Part model, mm, in its own coordinate system. Face numbers are marked on the shaded views. A direction names the side the tool comes from. Coordinates: 2 decimals unless noted, no trailing zeros. Order: outer loops, then holes, each group sorted by start corner. A loop starts at its lowest first (then second) coordinate and runs counter-clockwise, first axis right, second up. Notation, with made-up numbers: (66.25, 22) - (89.25, 22) arc R30 ccw to (89.25, 48) - close; hole circle Ø1 at (38, 72.5). An arc over 180 degrees is marked (long way). Use a Markdown table: item, result. Add a question column.
1) Saw through at A-A on x = 0. List the corners of the cut face in (y, z), then the cut area to 3 significant figures.
2) Drop flat-ended pins along their axis: P1, Ø1.5, axis at y = 41, z = 14.5, coming from the +X side; P2, Ø5.5, axis at x = 22, z = 7, coming from the +Y side; P3, Ø5.5, axis at x = -20, z = 9, coming from the +Y side. Give the stop position or say it passes through.
3) Two-plate mould, pull along Y, no slides. Class the marked faces 1, 2 and 3: +Y half, -Y half, draft (parallel to the pull), parting line (faces both ways), or undercut.
4) Saw through at B-B on y = 26.5. List the corners of the cut face in (x, z).
5) Saw through at C-C on z = 6. Count the separate pieces of the cut face and the enclosed holes in it, then the cut area to 3 significant figures.
6) Wall check: L1, parallel to X at y = 7.75, z = 15.3 (3 decimals); L2, parallel to X at y = 20.5, z = 14.75; L3, parallel to Y at x = 0, z = 9.75. Give the ranges that are in metal, low to high. Write a range as [from, to].
7) Tool access for the marked faces 4 and 5: list every direction of +Z, -Z, +X, -X, +Y, -Y with a clear straight run to the whole face (end or side of a thin tool).
```python
from build123d import *

# Parameters (mm, degrees)
SKETCH_1_R               = 6
EXTRUDE_1_DEPTH          = 18.3
CUT_EXTRUDE_1_DEPTH      = 38
SKETCH_3_R               = 2.15
CUT_EXTRUDE_2_DEPTH      = 74
CUT_EXTRUDE_START        = -74
SKETCH_5_W               = 10
SKETCH_5_H               = 40.552439024
CUT_EXTRUDE_3_DEPTH      = 156.521752466
CUT_EXTRUDE_4_DEPTH      = 40
SKETCH_8_W               = 6
SKETCH_8_H               = 37.346305337
EXTRUDE_2_DEPTH          = 18.3
FILLET_2_R               = 3
FILLET_3_R               = 5
CUT_EXTRUDE_7_DEPTH      = 80
CUT_EXTRUDE_7_DEPTH_BACK = 40
SKETCH_12_R              = 1.525


with BuildPart() as part:
    # 草图1 → 凸台-拉伸1 (new body)
    with BuildSketch(Plane.XY):
        with BuildLine():
            Line((-8.281928864, 111.239451243), (-56, 56.65))
            Line((-56, 56.65), (-56, 0))
            Line((-56, 0), (56, 0))
            Line((56, 0), (56, 56.65))
            Line((56, 56.65), (8.281928864, 111.239451243))
            ThreePointArc((8.281928864, 111.239451243), (0, 115), (-8.281928864, 111.239451243))
        make_face()
        with Locations((0, 104)):
            Circle(SKETCH_1_R, mode=Mode.SUBTRACT)
    extrude(amount=EXTRUDE_1_DEPTH)

    # 草图2 → Cut-Extrude 1 (cut)
    with BuildSketch(Plane.XY.offset(18.3)):
        Polygon((15.622574059, 56.346305337), (56, 36.65), (56, 56.65), (30, 116.346305337), (-30, 116.346305337), (-56, 56.65), (-56, 36.65), (-15.622574059, 56.346305337), align=None)
    extrude(amount=-CUT_EXTRUDE_1_DEPTH, mode=Mode.SUBTRACT)

    # 草图3 → 切除-拉伸2 (cut)
    with BuildSketch(Plane.XY.offset(18.3)):
        with Locations((0, 51.346305337)):
            Circle(SKETCH_3_R)
        with Locations((43, 31.65)):
            Circle(SKETCH_3_R)
        with Locations((43, 5)):
            Circle(SKETCH_3_R)
        with Locations((-43, 5)):
            Circle(SKETCH_3_R)
        with Locations((-43, 31.65)):
            Circle(SKETCH_3_R)
        with Locations((0, 5)):
            Circle(SKETCH_3_R)
    extrude(amount=-CUT_EXTRUDE_2_DEPTH, mode=Mode.SUBTRACT)

    # 草图5 → Cut-Extrude 3 (cut)
    with BuildSketch(Plane.XY.offset(18.3).offset(CUT_EXTRUDE_START)):
        with Locations((53, 20.276219512)):
            Rectangle(SKETCH_5_W, SKETCH_5_H)
    cut_extrude_3 = extrude(amount=CUT_EXTRUDE_3_DEPTH, mode=Mode.SUBTRACT)

    # 镜向2: Cut-Extrude 3 across plane
    add(cut_extrude_3.mirror(Plane(origin=(0, 0, 0), x_dir=(0, 0, 1), z_dir=(1, 0, 0))), mode=Mode.SUBTRACT)

    # 草图7 → 切除-拉伸4 (cut)
    with BuildSketch(Plane(origin=(0, 0, 0), x_dir=(-1, 0, 0), z_dir=(0, 0, -1))):
        Polygon((-38, 34.304151485), (-38, 10), (38, 10), (38, 34.304151485), (11.263584603, 47.346305337), (-11.263584603, 47.346305337), align=None)
    extrude(amount=-CUT_EXTRUDE_4_DEPTH, mode=Mode.SUBTRACT)

    # 草图8 → 凸台-拉伸2 (add)
    with BuildSketch(Plane(origin=(0, 0, 0), x_dir=(-1, 0, 0), z_dir=(0, 0, -1))):
        with Locations((0, 28.673152669)):
            Rectangle(SKETCH_8_W, SKETCH_8_H)
    extrude(amount=-EXTRUDE_2_DEPTH)

    # 圆角2
    fillet_2_edges = [part.edges().sort_by_distance(p)[0] for p in [
        (38, 34.304151485, 9.15),
        (11.263584603, 47.346305337, 9.15),
        (-11.263584603, 47.346305337, 9.15),
        (-38, 34.304151485, 9.15),
        (-38, 10, 9.15),
        (38, 10, 9.15),
        (3, 10, 9.15),
        (-3, 10, 9.15),
        (-3, 47.346305337, 9.15),
        (3, 47.346305337, 9.15),
    ]]
    fillet(fillet_2_edges, radius=FILLET_2_R)

    # 圆角3
    fillet_3_edges = [part.edges().sort_by_distance(p)[0] for p in [
        (-48, 40.552439024, 9.15),
        (-48, 0, 9.15),
        (15.622574059, 56.346305337, 9.15),
        (-15.622574059, 56.346305337, 9.15),
        (48, 40.552439024, 9.15),
        (48, 0, 9.15),
    ]]
    fillet(fillet_3_edges, radius=FILLET_3_R)

    # 草图12 → 切除-拉伸7 (cut, two sides: drawn at the far end of the back side and taken through both)
    with BuildSketch(Plane(origin=(0, 10, 0), x_dir=(1, 0, 0), z_dir=(0, 1, 0)).offset(-CUT_EXTRUDE_7_DEPTH_BACK)):
        with Locations(Location((-10, -15.3, 0), (0, 0, 90))):
            Circle(SKETCH_12_R)
        with Locations(Location((10, -15.3, 0), (0, 0, 90))):
            Circle(SKETCH_12_R)
    extrude(amount=CUT_EXTRUDE_7_DEPTH + CUT_EXTRUDE_7_DEPTH_BACK, mode=Mode.SUBTRACT)


solid = part.part
```
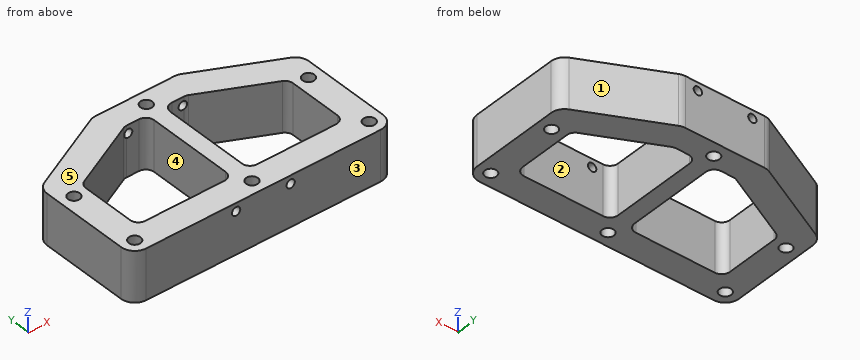
Results are:
| question | item | result |
|---|---|---|
| 1 | outline | (0, 0) - (2.85, 0) - (2.85, 18.3) - (0, 18.3) - close; (7.15, 0) - (49.2, 0) - (49.2, 18.3) - (7.15, 18.3) - close; (53.5, 0) - (56.35, 0) - (56.35, 18.3) - (53.5, 18.3) - close |
| 1 | area | 874 mm2 |
| 2 | P1 | x = 47.13 |
| 2 | P2 | y = 54.58 |
| 2 | P3 | y = 55.55 |
| 3 | face 1 | +Y half |
| 3 | face 2 | undercut |
| 3 | face 3 | -Y half |
| 4 | outline | (-48, 0) - (-38, 0) - (-38, 18.3) - (-48, 18.3) - close; (-3, 0) - (3, 0) - (3, 18.3) - (-3, 18.3) - close; (38, 0) - (48, 0) - (48, 18.3) - (38, 18.3) - close |
| 5 | separate pieces | 1 |
| 5 | enclosed holes | 8 |
| 5 | area | 2,540 mm2 |
| 6 | L1 | [-48, -11.525], [-8.475, 8.475], [11.525, 48] |
| 6 | L2 | [-48, -38], [-3, 3], [38, 48] |
| 6 | L3 | [0, 2.85], [7.15, 49.2], [53.5, 56.35] |
| 7 | face 4 | +Z, -Z |
| 7 | face 5 | +Z, +X, -X, +Y, -Y |
